from build123d import *

# Parameters (mm, degrees)
ESQUISSE3_W             = 14
ESQUISSE3_H             = 2
BOSS_EXTRU_1_DEPTH      = 10
BOSS_EXTRU_1_2_DEPTH    = 10
ESQUISSE4_W             = 9.2
ESQUISSE4_H             = 2
BOSS_EXTRU_2_DEPTH      = 14
BOSS_EXTRU_3_DEPTH      = 12
CONG_2_R                = 0.5
CONG_4_R                = 1
CONG_5_R                = 1
CONG_6_R                = 1
ESQUISSE6_W             = 23
ESQUISSE6_H             = 0.979911891
BOSS_EXTRU_4_DEPTH      = 12
CONG_8_R                = 0.5
ESQUISSE7_W             = 0.4
ESQUISSE7_H             = 10.548698827
ENL_V_MAT_EXTRU_1_DEPTH = 1.5


with BuildPart() as part:
    # Esquisse3 → Boss.-Extru.1 (new body)
    with BuildSketch(Plane(origin=(0, 0, 0), x_dir=(1, 0, 0), z_dir=(0, 1, 0))):
        with Locations((-7, 6.2)):
            Rectangle(ESQUISSE3_W, ESQUISSE3_H)
    extrude(amount=BOSS_EXTRU_1_DEPTH)



with BuildPart() as body_2:
    # Esquisse3 → Boss.-Extru.1 2 (new body)
    with BuildSketch(Plane(origin=(0, 0, 0), x_dir=(1, 0, 0), z_dir=(0, 1, 0))):
        with Locations((-7, -1)):
            Rectangle(ESQUISSE3_W, ESQUISSE3_H)
    extrude(amount=BOSS_EXTRU_1_2_DEPTH)


with BuildPart() as part_1:
    add(part.part)

    add(body_2.part)  # Boss.-Extru.2 merges body 2
    # Esquisse4 → Boss.-Extru.2 (add)
    with BuildSketch(Plane(origin=(0, 0, 0), x_dir=(0, 0, -1), z_dir=(1, 0, 0))):
        with Locations((2.6, -1)):
            Rectangle(ESQUISSE4_W, ESQUISSE4_H)
    extrude(amount=-BOSS_EXTRU_2_DEPTH)

    # Esquisse5 → Boss.-Extru.3 (add)
    with BuildSketch(Plane.XZ.offset(2)):
        Polygon((-14, 2), (-19, 2), (-19, 22.8), (-18.5, 22.8), (-18.5, 2.8), (4.5, 2.8), (4.5, 22.8), (5, 22.8), (5, 2), (0, 2), align=None)
    extrude(amount=-BOSS_EXTRU_3_DEPTH)

    # Congé2
    # the kernel refuses this fillet: 0.5 mm, written as the material it takes off along each edge
    with BuildSketch(Plane(origin=(-19, -3.25, 22.8), x_dir=(0, 0, -1), z_dir=(0, 1, 0)), Plane(origin=(-18.5, -3.25, 22.8), x_dir=(-1, 0, 0), z_dir=(0, 1, 0)), Plane(origin=(4.5, -3.25, 22.8), x_dir=(0, 0, -1), z_dir=(0, 1, 0)), Plane(origin=(5, -3.25, 22.8), x_dir=(-1, 0, 0), z_dir=(0, 1, 0))) as cong_2_piece_1:
        with BuildLine():
            CenterArc((CONG_2_R, -CONG_2_R), CONG_2_R, 90, 90)
            Line((0, -CONG_2_R), (0, 0))
            Line((0, 0), (CONG_2_R, 0))
        make_face()
    extrude(amount=14.5, mode=Mode.SUBTRACT)

    # Congé4
    cong_4_edges = [part_1.edges().sort_by_distance(p)[0] for p in [
        (-19, 4, 2),
    ]]
    fillet(cong_4_edges, radius=CONG_4_R)

    # Congé5
    cong_5_edges = [part_1.edges().sort_by_distance(p)[0] for p in [
        (5, 4, 2),
    ]]
    fillet(cong_5_edges, radius=CONG_5_R)

    # Congé6
    cong_6_edges = [part_1.edges().sort_by_distance(p)[0] for p in [
        (-14, 4, 2),
        (0, 4, 2),
    ]]
    fillet(cong_6_edges, radius=CONG_6_R)

    # Esquisse6 → Boss.-Extru.4 (add)
    with BuildSketch(Plane(origin=(0, -2, 0), x_dir=(-1, 0, 0), z_dir=(0, -1, 0))):
        with Locations((7, -6.745764799)):
            Rectangle(ESQUISSE6_W, ESQUISSE6_H)
    extrude(amount=-BOSS_EXTRU_4_DEPTH)

    # Congé8
    cong_8_edges = [part_1.edges().sort_by_distance(p)[0] for p in [
        (-18.5, 4, 6.255808853),
        (4.5, 4, 6.255808853),
        (-18.5, 4, 2.8),
        (4.5, 4, 2.8),
    ]]
    fillet(cong_8_edges, radius=CONG_8_R)

    # Esquisse7 → Enlèv. mat.-Extru.1 (cut)
    with BuildSketch(Plane.XY.offset(7.235720744)):
        with Locations((-18.05, 3.759681921)):
            Rectangle(ESQUISSE7_W, ESQUISSE7_H)
        with Locations((-17.05, 3.759681921)):
            Rectangle(ESQUISSE7_W, ESQUISSE7_H)
        with Locations((-16.05, 3.759681921)):
            Rectangle(ESQUISSE7_W, ESQUISSE7_H)
        with Locations((-15.05, 3.759681921)):
            Rectangle(ESQUISSE7_W, ESQUISSE7_H)
        with Locations((-14.05, 3.759681921)):
            Rectangle(ESQUISSE7_W, ESQUISSE7_H)
        with Locations((-13.05, 3.759681921)):
            Rectangle(ESQUISSE7_W, ESQUISSE7_H)
        with Locations((-12.05, 3.759681921)):
            Rectangle(ESQUISSE7_W, ESQUISSE7_H)
        with Locations((-11.05, 3.759681921)):
            Rectangle(ESQUISSE7_W, ESQUISSE7_H)
        with Locations((-10.05, 3.759681921)):
            Rectangle(ESQUISSE7_W, ESQUISSE7_H)
        with Locations((-9.05, 3.759681921)):
            Rectangle(ESQUISSE7_W, ESQUISSE7_H)
        with Locations((-8.05, 3.759681921)):
            Rectangle(ESQUISSE7_W, ESQUISSE7_H)
        with Locations((-7.05, 3.759681921)):
            Rectangle(ESQUISSE7_W, ESQUISSE7_H)
        with Locations((-6.05, 3.759681921)):
            Rectangle(ESQUISSE7_W, ESQUISSE7_H)
        with Locations((-5.05, 3.759681921)):
            Rectangle(ESQUISSE7_W, ESQUISSE7_H)
        with Locations((-4.05, 3.759681921)):
            Rectangle(ESQUISSE7_W, ESQUISSE7_H)
        with Locations((-3.05, 3.759681921)):
            Rectangle(ESQUISSE7_W, ESQUISSE7_H)
        with Locations((-2.05, 3.759681921)):
            Rectangle(ESQUISSE7_W, ESQUISSE7_H)
        with Locations((-1.05, 3.759681921)):
            Rectangle(ESQUISSE7_W, ESQUISSE7_H)
        with Locations((-0.05, 3.759681921)):
            Rectangle(ESQUISSE7_W, ESQUISSE7_H)
        with Locations((0.95, 3.759681921)):
            Rectangle(ESQUISSE7_W, ESQUISSE7_H)
        with Locations((1.95, 3.759681921)):
            Rectangle(ESQUISSE7_W, ESQUISSE7_H)
        with Locations((2.95, 3.759681921)):
            Rectangle(ESQUISSE7_W, ESQUISSE7_H)
        with Locations((3.95, 3.759681921)):
            Rectangle(ESQUISSE7_W, ESQUISSE7_H)
    extrude(amount=-ENL_V_MAT_EXTRU_1_DEPTH, mode=Mode.SUBTRACT)


solid = part_1.part
Input: part model. Units: mm. Frame: model coordinates. A direction names the side the tool comes from. Give positions to 0.01 mm unless a question says otherwise; leave off trailing zeros. Loops run counter-clockwise (first coordinate to the right, second up) from the corner with the lowest first, then second, coordinate; pieces in that order, holes last. Notation, with made-up numbers: M -28,89 L 7,89 A18 cw 7,97 Z; hole C 84,60 d1. An arc over 180 degrees is marked long. Use one line per item in the form item = value.
1. Section query A-A, the plane z = 13. Return the cut outline in (x, y).
Numbers:
outline = M -19,-2 L -18.5,-2 L -18.5,10 L -19,10 Z; M 4.5,-2 L 5,-2 L 5,10 L 4.5,10 Z
2. First-contact query: pin 1 (8 mm diameter, centred on x = -16.5, z = -2, fed in from -Y); pin 2 (1.5 mm diameter, centred on x = -16, y = 0, fed in from -Z); pin 3 (3 mm diameter, centred on x = -9.5, y = 6.5, fed in from +Z). Flat tips, straight axial feed; report the tip coordinate or a pass-through.
Numbers:
pin_1 = -2
pin_2 = 2
pin_3 = 7.24
3. Pull-direction query (Y, two-part tool) for faces 1 (the face through (0.75, 4, 7)), 2 (the face through (-7, 4, -7.2)); classes: released by +Y, released by -Y, zero draft, split by the parting line, or undercut.
Numbers:
face_1 = undercut
face_2 = zero draft
4. Line query: L1, parallel to Z at x = -0.5, y = 6; L2, parallel to Z at x = -15.75, y = 1; L3, parallel to Z at x = -2.75, y = -1. Output: solid intervals per line, ascending.
Numbers:
L1 = -7.2 to -5.2, 0 to 2.8, 6.26 to 7.24
L2 = 2 to 2.8, 6.26 to 7.24
L3 = -7.2 to 2.8, 6.26 to 7.24
5. Section query B-B, the plane y = 1.25. Count the separate pieces of the cut face and the enclosed holes in it, and give its area (3 significant figures).
Numbers:
separate_pieces = 24
enclosed_holes = 0
area = 109 mm²
6. Section query C-C, the plane z = -2.5. Return the cut outline in (x, y), and give its area (3 significant figures).
Numbers:
outline = M -14,-2 L 0,-2 L 0,0 L -14,0 Z
area = 28.0 mm²
7. Reachability of faces 3 (the face through (-7, 5, 0)), 4 (the face through (4.699, 4.084, 2.285)), 5 (the face through (-17, 4, 2)), 6 (the face through (-15.85, 4, 7)) from +Z, -Z, +X, -X, +Y, -Y: full face, straight path, thin tool, end or side. Return the list, or none.
Numbers:
face_3 = +X, -X, +Y
face_4 = -Z, +X, +Y, -Y
face_5 = -Z, -X, +Y, -Y
face_6 = +Z
